Autodesk Inventor part; units mm, degrees
ref_plane "Work Plane2" through (0, 196.485, 0) normal (0, 1, 0) x (1, 0, 0)
ref_plane "Work Plane3" through (0, 166.485, 0) normal (0, 1, 0) x (1, 0, 0)
ref_plane "Work Plane5" through (0, 87.715, 0) normal (0, 1, 0) x (1, 0, 0)
sketch "Sketch1" plane through (0, 0, 0) normal (0, 1, 0) x (-1, 0, 0)
  circle A0 centre (0, 0) radius 10
  dimension "d2" = 20
extrude "Extrusion1" add sketch "Sketch1" along normal blind 283
ref_plane "Work Plane1" through (0, 181.485, 0) normal (0, 1, 0) x (1, 0, 0)
ref_plane "Work Plane2" through (0, 196.485, 0) normal (0, 1, 0) x (1, 0, 0)
ref_plane "Work Plane3" through (0, 166.485, 0) normal (0, 1, 0) x (1, 0, 0)
sketch "Sketch2" plane through (0, 196.485, 0) normal (0, 1, 0) x (1, 0, 0)
  circle A0 centre (0, 0) radius 12.5
  line L0 (-11.3632, -5.2083) -> (0, -30)
  line L1 (0, -30) -> (11.3632, -5.2083)
  dimension "d6" = 25
  dimension "d7" = 30
extrude "Extrusion2" add sketch "Sketch2" along normal mid plane 10
sketch "Sketch4" plane through (0, 166.485, 0) normal (0, 1, 0) x (1, 0, 0)
  circle A0 centre (0, 0) radius 12.5
  line L0 (0, -30) -> (11.3632, -5.2083) construction
  line L1 (0, 0) -> (0, -30) construction
  line L2 (0, 0) -> (-28.1908, 10.2606) construction
  line L3 (-1.0078, 12.4593) -> (-28.1908, 10.2606)
  line L4 (-28.1908, 10.2606) -> (-8.7807, -8.8966)
  point P0 (0, -12.5552)
  point P1 (0, -12.5)
  point P2 (6.0758, -7.9426)
  point P3 (10.4096, -7.2889)
  point P4 (0, -12.5552)
  dimension "d10" = 25
  dimension "d12" = 30
  dimension "d19" = 250
extrude "Extrusion3" add sketch "Sketch4" along normal mid plane 10
ref_plane "Work Plane4" through (0, 72.715, 0) normal (0, 1, 0) x (1, 0, 0)
ref_plane "Work Plane5" through (0, 87.715, 0) normal (0, 1, 0) x (1, 0, 0)
ref_plane "Work Plane6" through (0, 57.715, 0) normal (0, 1, 0) x (1, 0, 0)
fillet "Fillet1" radius 5 2 edges at (-28.1908, 166.485, -10.2606) (0, 196.485, 30)
sketch "Sketch5" plane through (0, 87.715, 0) normal (0, 1, 0) x (1, 0, 0)
  circle A0 centre (0, 0) radius 12.5
  arc A1 (-4.5453, -20.0833) -> (4.5453, -20.0833) centre (0, -18) ccw
  line L0 (0, 0) -> (0, -18) construction
  line L1 (0, 0) -> (-5.2094, -29.5442) construction
  line L2 (-5.2094, -29.5442) -> (-12.095, -3.156)
  line L3 (-5.2094, -29.5442) -> (10.2862, -7.1024)
  dimension "d21" = 25
  dimension "d22" = 10
  dimension "d23" = 30
extrude "Extrusion4" add sketch "Sketch5" along normal mid plane 10
sketch "Sketch6" plane through (0, 57.715, 0) normal (0, 1, 0) x (1, 0, 0)
  circle A0 centre (0, 0) radius 12.5
  line L0 (-8.7807, -8.8966) -> (-20.4267, 2.5977)
  line L1 (8.7807, -8.8966) -> (28.1908, 10.2606)
  line L2 (28.1908, 10.2606) -> (1.0078, 12.4593)
  line L3 (0, 0) -> (0, -18) construction
  line L4 (28.1908, 10.2606) -> (0, 0) construction
  dimension "d26" = 25
  dimension "d27" = 18
  dimension "d28" = 30
  dimension "d29" = 250
extrude "Extrusion5" add sketch "Sketch6" along normal mid plane 10
fillet "Fillet2" radius 5 2 edges at (28.1908, 57.715, -10.2606) (-5.2094, 87.715, 29.5442)
sketch "Sketch7" plane through (0, 0, 0) normal (0, -1, 0) x (1, 0, 0)
  circle A0 centre (0, 0) radius 15
  circle A1 centre (0, 0) radius 30
  dimension "d33" = 30
  dimension "d34" = 60
extrude "Extrusion6" add sketch "Sketch7" against normal blind 8
extrude "Extrusion7" add sketch "Sketch7" against normal blind 10 contours A0
sketch "Sketch8" plane through (0, 0, 0) normal (0, -1, 0) x (1, 0, 0)
  line L0 (15, -2.5) -> (-15, -2.5)
  line L1 (-15, -2.5) -> (-15, 2.5)
  line L2 (-15, 2.5) -> (15, 2.5)
  line L3 (15, 2.5) -> (15, -2.5)
  line L4 (15, -2.5) -> (-15, 2.5) construction
  line L5 (-15, -2.5) -> (15, 2.5) construction
  circle A0 centre (0, 0) radius 22.5
  circle A1 centre (0, 0) radius 5
  point P0 (-22.5, 0)
  point P1 (11.25, -19.4856)
  point P2 (11.25, 19.4856)
  point P3 (4.3301, 2.5)
  point P4 (-4.3301, 2.5)
  point P5 (-4.3301, -2.5)
  point P6 (4.3301, -2.5)
  dimension "d43" = 45
  dimension "d41" = 360
  dimension "d44" = 5
  dimension "d45" = 30
  dimension "d48" = 10
extrude "Extrusion8" cut sketch "Sketch8" against normal blind 5 contours L0 A1 L2 L3 | A1 L0 | L0 A1 L2 | L0 L1 L2 A1 | L2 A1
hole "Hole1" at (-22.5, 0, 0) at (11.25, 0, -19.4856) at (11.25, 0, 19.4856) direction (0, 1, 0) diameter 4.134 depth 5
ref_plane "Work Plane7" through (0, 31.76, 0) normal (0, 1, 0) x (1, 0, 0)
sketch "Sketch9" plane through (0, 31.76, 0) normal (0, 1, 0) x (1, 0, 0)
  circle A0 centre (0, 0) radius 17.5
  dimension "d57" = 35
extrude "Extrusion9" add sketch "Sketch9" along normal blind 3
properties part number "Wałek rozrządu"
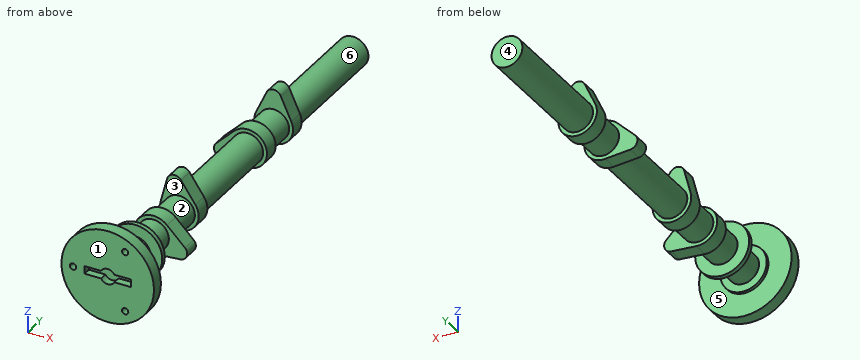
Build history of the part. All positions in model axes, mm. Face numbers are marked on the shaded views. A direction names the side the tool comes from. Round coordinates to 2 decimals unless told otherwise and drop trailing zeros. Loops run counter-clockwise (first coordinate to the right, second up) from the corner with the lowest first, then second, coordinate; pieces in that order, holes last. Notation, with made-up numbers: (65, 25) -> (90, 25) arc R24 cw to (90, 35) -> close; hole circle Ø3 at (83.25, 76). An arc over 180 degrees is marked (long way). One line per item, written item: value. Start each with the question number.
Q1. Probe line 1 along Y through (x, z) = (11, -6.5) (3 decimals); line 2 along Z through (x, y) = (11, 3); line 3 along Y through (x, z) = (-5.5, 9) (3 decimals). List the from-to ranges inside material, lowest first.
Q2. 3-axis set-ups, long thin cutter, end or side, ignore diameter. For the marked faces 1 and 2: which of +Z, -Z, +X, -X, +Y, -Y reach the whole face in a straight line?
Q3. Drop flat-ended pins along their axis: pin 1 Ø4 at (x, y) = (10.5, 1.5) entering from +Z; pin 2 Ø1 at (x, z) = (-13.5, 0) entering from +Y (3 decimals); pin 3 Ø3.5 at (x, z) = (-22.5, 0) entering from -Y. Give the stop position or say it passes through.
Q4. Cut at A-A on y = 244. List the corners of the cut face in (x, z).
Q5. Two-plate mould, pull along Y, no slides. Class the marked faces 3, 4, 5 and 6: released by +Y, released by -Y, zero draft, split by the parting line, or undercut.
Computed:
1. line 1: 0 to 10, 31.76 to 34.76, 52.715 to 62.715
1. line 2: -27.91 to -21.54, -17.43 to -2.5, 2.5 to 17.43, 21.54 to 27.91
1. line 3: 0 to 10, 31.76 to 34.76, 52.715 to 62.715, 82.715 to 92.715, 161.485 to 171.485, 191.485 to 201.485
2. face 1: +Z, -Z, +X, -X, -Y
2. face 2: none
3. pin 1: z = 28.77
3. pin 2: y = 171.485
3. pin 3: y = 5
4. outline: circle Ø20 at (0, 0)
5. face 3: undercut
5. face 4: released by +Y
5. face 5: undercut
5. face 6: zero draft
